Part print with two shaded views. Sizes in mm from the minimum x, y, z corner. A direction names the side the tool comes from. Give positions to 0.01 mm unless a question says otherwise; leave off trailing zeros. Write each loop counter-clockwise with the first axis right and the second up, starting at its lowest first coordinate (ties: lowest second). Pieces come first, ordered by that corner, then holes.
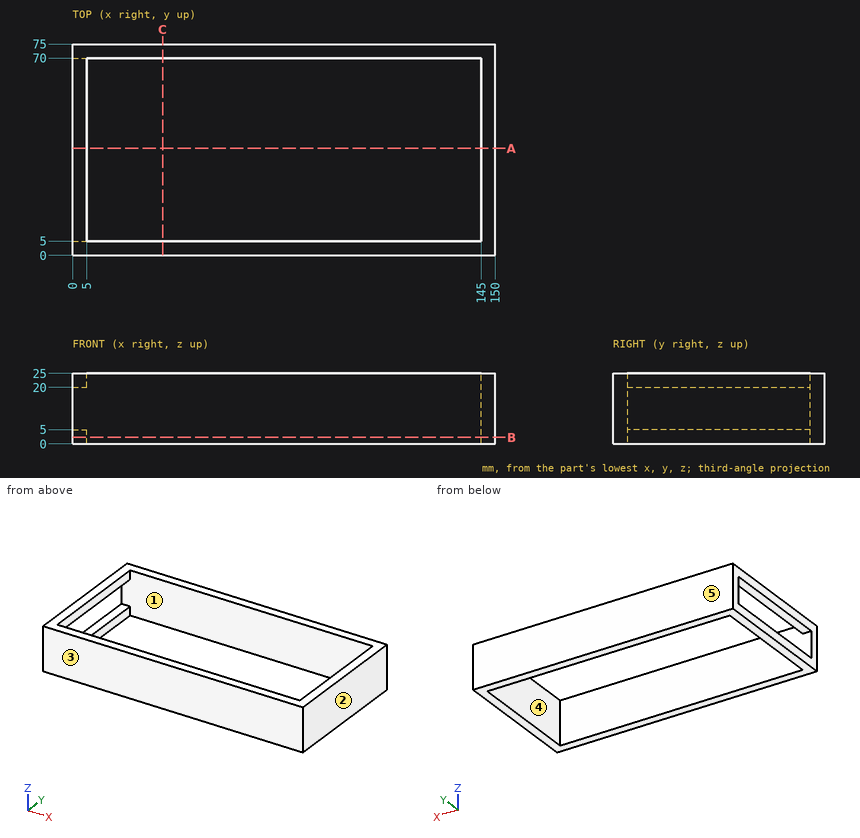
1) Drill centre lines: L1, parallel to Y at x = 28.5, z = 19.5; L2, parallel to X at y = 63.5, z = 21.75; L3, parallel to X at y = 35, z = 5.5. Where is each one in solid material? Low to high.
Check result:
L1: y = 0 to 5, 70 to 75
L2: x = 0 to 5, 145 to 150
L3: x = 145 to 150
2) Saw through at A-A (y = 38). Write the cut outline in (x, z), and give its area (3 significant figures).
Check result:
outline: (0, 0) - (5, 0) - (5, 5) - (0, 5) - close; (0, 20) - (5, 20) - (5, 25) - (0, 25) - close; (145, 0) - (150, 0) - (150, 25) - (145, 25) - close
area: 175 mm2
3) Flat gauge pins, fed straight in: P1, Ø5, axis at y = 54.5, z = 10, coming from the -X side; P2, Ø1, axis at x = 118.5, z = 18, coming from the -Y side. Where does each tip first touch, or does it go through?
Check result:
P1: stops at x = 145
P2: stops at y = 0
4) Saw through at B-B (z = 2.25). Write the cut outline in (x, y).
Check result:
outline: (0, 0) - (150, 0) - (150, 75) - (0, 75) - close; hole (5, 5) - (145, 5) - (145, 70) - (5, 70) - close
5) Mould opens along X. For the marked faces 1, 2 and 3 say: +X half, -X half, draft (parallel to the pull), parting line (faces both ways), or undercut.
Check result:
face 1: undercut
face 2: +X half
face 3: draft
6) Saw through at C-C (x = 32). Write the cut outline in (y, z), and give its area (3 significant figures).
Check result:
outline: (0, 0) - (5, 0) - (5, 25) - (0, 25) - close; (70, 0) - (75, 0) - (75, 25) - (70, 25) - close
area: 250 mm2
7) 3-axis set-ups, long thin cutter, end or side, ignore diameter. For the marked faces 4 and 5: which of +Z, -Z, +X, -X, +Y, -Y reach the whole face in a straight line?
Check result:
face 4: +Z, -Z
face 5: +Z, -Z, +X, -X, +Y
